from build123d import *

# Parameters (mm, degrees)
F0_W     = 101.6
F0_H     = 76.2
F1_DEPTH = 25.4
F2_R     = 6.35
F3_DEPTH = 25.4
F4_W     = 25.4
F4_H     = 38.1
F6_W     = 23.010891
F6_H     = 6.35
F8_SIZE  = 2.54
F9_R     = 2.54


with BuildPart() as f1:
    # F0 (on Top) → F1 (new body)
    with BuildSketch(Plane.XY):
        Rectangle(F0_W, F0_H)
    extrude(amount=F1_DEPTH)

    # F2 (on face) → F3 (cut)
    with BuildSketch(Plane.XY.offset(25.4)):
        with Locations((-38.1, 25.4)):
            Circle(F2_R)
        with Locations((38.1, 25.4)):
            Circle(F2_R)
        with Locations((38.1, -25.4)):
            Circle(F2_R)
        with Locations((-38.1, -25.4)):
            Circle(F2_R)
    extrude(amount=-F3_DEPTH, mode=Mode.SUBTRACT)

    # F4 (on Front) → F5 (revolve)
    with BuildSketch(Plane.XZ):
        with Locations((-12.7, 44.45)):
            Rectangle(F4_W, F4_H)
    revolve(axis=Axis((0, 0, 44.45), (0, 0, -1)))

    # F6 (on Front) → F7 (revolve, cut)
    with BuildSketch(Plane.XZ):
        with Locations((-30.555445, 41.275)):
            Rectangle(F6_W, F6_H)
    revolve(axis=Axis((0, 0, 63.5), (0, 0, -1)), mode=Mode.SUBTRACT)

    # F8
    f8_edges = [f1.edges().sort_by_distance(p)[0] for p in [
        (0, -38.1, 25.4),
        (50.8, 0, 25.4),
        (-50.8, 0, 25.4),
        (0, 38.1, 25.4),
    ]]
    chamfer(f8_edges, length=F8_SIZE)

    # F9
    f9_edges = [f1.edges().sort_by_distance(p)[0] for p in [
        (25.4, 0, 63.5),
        (25.4, 0, 25.4),
    ]]
    fillet(f9_edges, radius=F9_R)


solid = f1.part
Part model, mm, in its own coordinate system. A direction names the side the tool comes from. Give positions to 0.01 mm unless a question says otherwise; leave off trailing zeros. Write each loop counter-clockwise with the first axis right and the second up, starting at its lowest first coordinate (ties: lowest second). Pieces come first, ordered by that corner, then holes.
1) Cut at A-A on x = -38.1. Write the cut outline in (y, z), then the cut area to 3 significant figures.
Resolved:
outline: (-38.1, 0) - (-31.75, 0) - (-31.75, 25.4) - (-35.56, 25.4) - (-38.1, 22.86) - close; (-19.05, 0) - (19.05, 0) - (19.05, 25.4) - (-19.05, 25.4) - close; (31.75, 0) - (38.1, 0) - (38.1, 22.86) - (35.56, 25.4) - (31.75, 25.4) - close
area: 1,280 mm2
2) Cut at C-C on y = 0. Write the cut outline in (x, z).
Resolved:
outline: (-50.8, 0) - (50.8, 0) - (50.8, 22.86) - (48.26, 25.4) - (27.94, 25.4) arc R2.54 cw to (25.4, 27.94) - (25.4, 38.1) - (19.05, 38.1) - (19.05, 44.45) - (25.4, 44.45) - (25.4, 60.96) arc R2.54 ccw to (22.86, 63.5) - (-22.86, 63.5) arc R2.54 ccw to (-25.4, 60.96) - (-25.4, 44.45) - (-19.05, 44.45) - (-19.05, 38.1) - (-25.4, 38.1) - (-25.4, 27.94) arc R2.54 cw to (-27.94, 25.4) - (-48.26, 25.4) - (-50.8, 22.86) - close
3) Two-plate mould, pull along Y, no slides. Class faces 4 (the face through (33.06, -29.26, 12.88)), 5 (the face through (-1, 38.1, 11)), 6 (the face through (0, 0, 63.5)): released by +Y, released by -Y, zero draft, split by the parting line, or undercut.
Resolved:
face 4: undercut
face 5: released by +Y
face 6: zero draft
4) Probe L1, parallel to X at y = 25, z = 20; L2, parallel to Y at x = 38.1, z = 18; L3, parallel to Y at x = -34.5, z = 21.5. List the from-to ranges inside material, lowest first.
Resolved:
L1: x = -50.8 to -44.44, -31.76 to 31.76, 44.44 to 50.8
L2: y = -38.1 to -31.75, -19.05 to 19.05, 31.75 to 38.1
L3: y = -38.1 to -30.63, -20.17 to 20.17, 30.63 to 38.1
5) Cut at D-D on x = 0. Write the cut outline in (y, z).
Resolved:
outline: (-38.1, 0) - (38.1, 0) - (38.1, 22.86) - (35.56, 25.4) - (27.94, 25.4) arc R2.54 cw to (25.4, 27.94) - (25.4, 38.1) - (19.05, 38.1) - (19.05, 44.45) - (25.4, 44.45) - (25.4, 60.96) arc R2.54 ccw to (22.86, 63.5) - (-22.86, 63.5) arc R2.54 ccw to (-25.4, 60.96) - (-25.4, 44.45) - (-19.05, 44.45) - (-19.05, 38.1) - (-25.4, 38.1) - (-25.4, 27.94) arc R2.54 cw to (-27.94, 25.4) - (-35.56, 25.4) - (-38.1, 22.86) - close
6) Pin check, flat tips, straight feed: pin 1 (3 mm diameter, centred on y = -10, z = 36, fed in from -X); pin 2 (3 mm diameter, centred on y = -2.5, z = 31.5, fed in from -X); pin 3 (8 mm diameter, centred on x = 35, y = 8.5, fed in from +Z). Stop position of each tip, or through.
Resolved:
pin 1: stops at x = -23.94
pin 2: stops at x = -25.38
pin 3: stops at z = 25.4
7) Which spindle directions (+Z, -Z, +X, -X, +Y, -Y) get a long thin tool onto all of the face, cutting with end or side? Do faces 1 (the face through (-49.51, -0.53, 24.15)), 2 (the face through (-4, 19, 44.45)), 3 (the face through (31, 0, 25.4)). Say none if no direction does.
Resolved:
face 1: +Z, -X, +Y, -Y
face 2: none
face 3: +Z
8) Cut at B-B on z = 5. Write the cut outline in (x, y).
Resolved:
outline: (-50.8, -38.1) - (50.8, -38.1) - (50.8, 38.1) - (-50.8, 38.1) - close; hole circle Ø12.7 at (-38.1, -25.4); hole circle Ø12.7 at (-38.1, 25.4); hole circle Ø12.7 at (38.1, -25.4); hole circle Ø12.7 at (38.1, 25.4)
